Read the model definition and answer for the solid it produces. Units are mm, in the model's axes. A direction names the side the tool comes from. Coordinates: 2 decimals unless noted, no trailing zeros. Loops run counter-clockwise (first coordinate to the right, second up) from the corner with the lowest first, then second, coordinate; pieces in that order, holes last. Notation, with made-up numbers: M 53,87.25 L 57,87.25 A14 ccw 57,112.25 Z; hole C 17.5,47.5 d10. An arc over 180 degrees is marked long. Put each result on its own line as item: value.
from build123d import *

# Parameters (mm, degrees)
BOSS_EXTRUDE1_DEPTH      = 50.8
BOSS_EXTRUDE1_DEPTH_BACK = 50.8
SKETCH2_R                = 5.5499
CHAMFER1_SIZE            = 0.9525
CUT_EXTRUDE1_DEPTH       = 52.402750705
CUT_EXTRUDE1_DEPTH_BACK  = 52.402750705
SKETCH5_W                = 1.5875
SKETCH5_H                = 1.5875


with BuildPart() as part:
    # Sketch2 → Boss-Extrude1 (new, two sides: drawn at the far end of the back side and taken through both)
    with BuildSketch(Plane(origin=(0, 0, 0), x_dir=(0, 0, -1), z_dir=(1, 0, 0)).offset(-BOSS_EXTRUDE1_DEPTH_BACK)):
        Circle(SKETCH2_R)
    extrude(amount=BOSS_EXTRUDE1_DEPTH + BOSS_EXTRUDE1_DEPTH_BACK)

    # Chamfer1
    chamfer1_edges = [part.edges().sort_by_distance(p)[0] for p in [
        (-50.8, 0, 5.5499),
        (50.8, 0, 5.5499),
    ]]
    chamfer(chamfer1_edges, length=CHAMFER1_SIZE)

    # Sketch5 → Cut-Extrude1 (cut, two sides: drawn at the far end of the back side and taken through both)
    with BuildSketch(Plane.XY.offset(-CUT_EXTRUDE1_DEPTH_BACK)):
        with Locations((-50.00625, 0)):
            Rectangle(SKETCH5_W, SKETCH5_H)
        with Locations((50.00625, 0)):
            Rectangle(SKETCH5_W, SKETCH5_H)
    extrude(amount=CUT_EXTRUDE1_DEPTH + CUT_EXTRUDE1_DEPTH_BACK, mode=Mode.SUBTRACT)


solid = part.part
1) Which of the six approach directions +Z, -Z, +X, -X, +Y, -Y give full straight-line access (tool end or side, diameter ignored) to faces 4 (the flat face through (49.212, 0, 0)), 5 (the flat face through (-50, 0.794, 0)), 6 (the conical face through (50.648, -4.749, 0.095))?
Answer list:
face 4: +Z, -Z, +X
face 5: +Z, -Z, -X
face 6: +X, -Y
2) Find section A-A, the plane x = -18. Write down the section's boundary in (y, z), plus the area to 3 significant figures.
Answer list:
outline: C 0,0 d11.1
area: 96.8 mm^2
3) Given pin 1 Ø0.8 at (y, z) = (0, -2) entering from -X; pin 2 Ø0.5 at (x, z) = (-50.5, 0.5) entering from -Y; pin 3 Ø1.3 at (x, z) = (49.5, 2.5) entering from +Y, each flat-ended and moving along its own axis, determine where each tip first touches the part or whether it passes through.
Answer list:
pin 1: stops at x = -49.21
pin 2: stops at y = -5.12
pin 3: stops at y = 5.23
4) Straight lines are drawn through the part: line 1 (Z direction, x = 29.5, y = 0.25); line 2 (X direction, y = 0.5, z = -0.25); line 3 (X direction, y = -4.5, z = 1). For each, find the intervals that lie inside material, in ascending order. Write a range as [from, to].
Answer list:
line 1: z = [-5.54, 5.54]
line 2: x = [-49.21, 49.21]
line 3: x = [-50.79, 50.79]
5) Determine the mould class of faces 1 (the conical face through (-50.648, 4.749, -0.095)), 2 (the flat face through (-50, -0.794, 0)), 3 (the flat face through (-50.8, -2, 0)) for opening direction Y: released by +Y, released by -Y, zero draft, split by the parting line, or undercut.
Answer list:
face 1: released by +Y
face 2: undercut
face 3: zero draft
